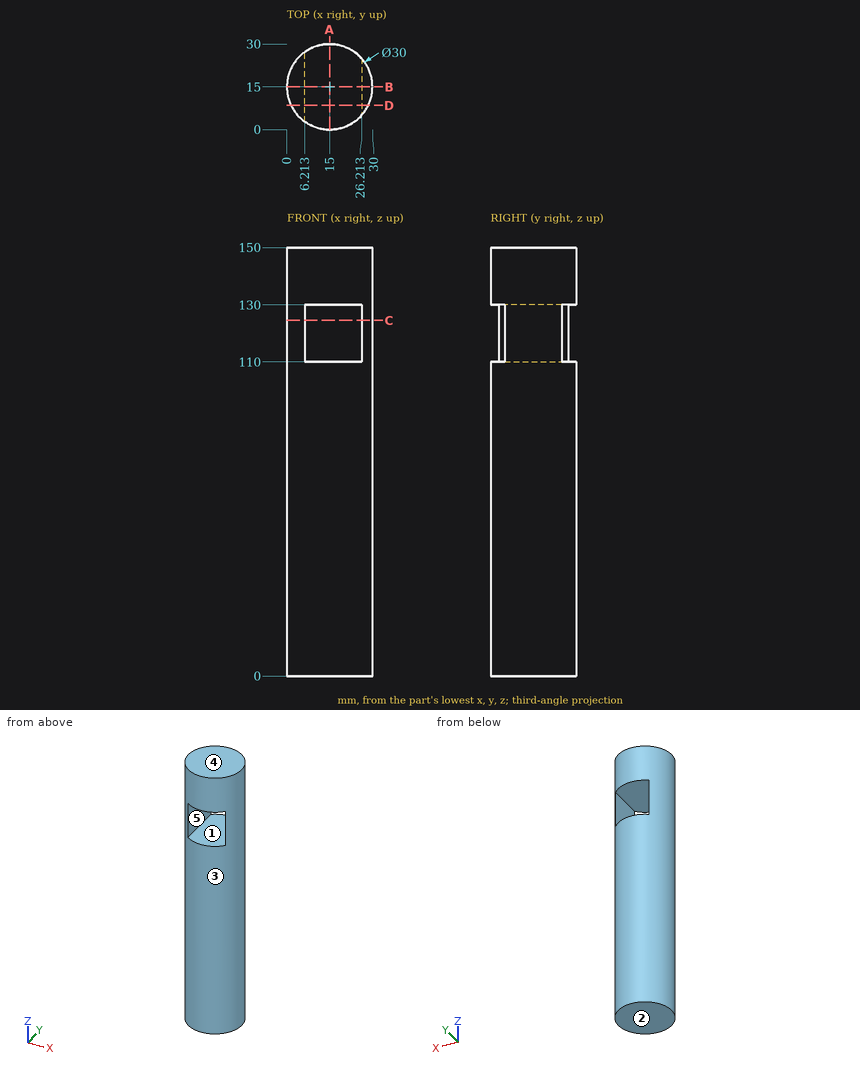
Drawing for the job (mm, zero at the part's lowest x, y, z). A direction names the side the tool comes from. Round coordinates to 2 decimals unless told otherwise and drop trailing zeros. Write each loop counter-clockwise with the first axis right and the second up, starting at its lowest first coordinate (ties: lowest second). Pieces come first, ordered by that corner, then holes. Notation, with made-up numbers: M 73.25,14.25 L 85.25,14.25 A29 ccw 85.25,49.25 Z; hole C 31,-35 d1. An arc over 180 degrees is marked long. Answer as a JSON object with one key per item and string values. Group by question number.
(1) Cut at C-C (z = 124.5). Give the cut face in (x, y).
(2) Drill centre lines: L1, parallel to Z at x = 20.5, y = 14; L2, parallel to Y at x = 15.75, z = 132.5; L3, parallel to X at y = 14.75, z = 38.5. Where is each one in solid material? Low to high.
(3) Flat gauge pins, fed straight in: pin 1 (6 mm diameter, centred on y = 9.5, z = 23.5, fed in from +X); pin 2 (2 mm diameter, centred on y = 20.5, z = 50, fed in from -X). Where does each tip first touch, or does it go through?
(4) Mould opens along X. For the marked faces 3, 4 and 5 say: pulls with the +X half, pulls with the -X half, needs draft (parallel to the pull), parting line crosses it, or undercut.
(5) Cut at A-A (x = 15). Give the cut face in (y, z), and give its area (3 significant figures).
(6) Cut at B-B (y = 15). Give the cut face in (x, z).
(7) Which spindle directions (+Z, -Z, +X, -X, +Y, -Y) get a long thin tool onto all of the face, cutting with end or side? Do the marked faces 1 and 2. Say none if no direction does.
(8) Cut at D-D (y = 8.5). Give the cut face in (x, z), and give its area (3 significant figures).
Responses:
{
 "1": {"outline": "M 6.21,2.84 L 6.21,27.16 A15 ccw Z; M 26.21,5.04 A15 ccw 26.21,24.96 Z"},
 "2": {"L1": "z = 0 to 110, 130 to 150", "L2": "y = 0.02 to 29.98", "L3": "x = 0 to 30"},
 "3": {"pin 1": "stops at x = 29.79", "pin 2": "stops at x = 0.69"},
 "4": {"face 3": "parting line crosses it", "face 4": "needs draft", "face 5": "undercut"},
 "5": {"outline": "M 0,0 L 30,0 L 30,110 L 0,110 Z; M 0,130 L 30,130 L 30,150 L 0,150 Z", "area": "3,900 mm2"},
 "6": {"outline": "M 0,0 L 30,0 L 30,150 L 0,150 Z; hole M 6.21,110 L 26.21,110 L 26.21,130 L 6.21,130 Z"},
 "7": {"face 1": "+Y, -Y", "face 2": "-Z, +X, -X, +Y, -Y"},
 "8": {"outline": "M 1.48,0 L 28.52,0 L 28.52,150 L 1.48,150 Z; hole M 6.21,110 L 26.21,110 L 26.21,130 L 6.21,130 Z", "area": "3,660 mm2"}
}
